Verification items for the finished model (mm, model axes). A direction names the side the tool comes from. Round coordinates to 2 decimals unless told otherwise and drop trailing zeros. Write each loop counter-clockwise with the first axis right and the second up, starting at its lowest first coordinate (ties: lowest second). Pieces come first, ordered by that corner, then holes. Notation, with made-up numbers: (52.5, 89) - (78.5, 89) arc R9 ccw to (78.5, 98) - close; hole circle Ø3 at (20.5, 38). An arc over 180 degrees is marked (long way). Answer as a JSON object with one key per item and string values.
```python
from build123d import *

# Parameters (mm, degrees)
SKETCH_2_W             = 6.925315878
SKETCH_2_H             = 1.1
CUT_EXTRUDE_1_DEPTH    = 11.1
HOLE_WIZARD_M8_1_D     = 6.8
HOLE_WIZARD_M8_1_DEPTH = 19.75
HOLE_WIZARD_M8_1_TIP   = 2.042926105
HOLE_WIZARD_M8_2_D     = 6.8
HOLE_WIZARD_M8_2_DEPTH = 19.75
HOLE_WIZARD_M8_2_TIP   = 2.042926105
CHAMFER_1_SIZE         = 0.2


with BuildPart() as part:
    # 草图1 → 旋转1 (revolve)
    with BuildSketch(Plane.XY):
        Polygon((0, 0), (6, 0), (6, 11.1), (8, 11.1), (8, 13.1), (5, 13.1), (5, 44), (0, 44), align=None)
    revolve(axis=Axis((0, -1000, 0), (0, 1, 0)))

    # 草图2 → 切除-拉伸1 (cut)
    with BuildSketch(Plane.XZ):
        with Locations((0, -5.45)):
            Rectangle(SKETCH_2_W, SKETCH_2_H)
        with Locations((0, 5.45)):
            Rectangle(SKETCH_2_W, SKETCH_2_H)
    extrude(amount=-CUT_EXTRUDE_1_DEPTH, mode=Mode.SUBTRACT)

    # M8 螺纹孔1
    with Locations(Plane(origin=(0, 44, 0), x_dir=(1, 0, 0), z_dir=(0, 1, 0))):
        with Locations((0, 0)):
            Hole(HOLE_WIZARD_M8_1_D / 2, depth=HOLE_WIZARD_M8_1_DEPTH)
            with Locations((0, 0, -(HOLE_WIZARD_M8_1_DEPTH + HOLE_WIZARD_M8_1_TIP / 2))):  # 118° drill point
                Cone(0, HOLE_WIZARD_M8_1_D / 2, HOLE_WIZARD_M8_1_TIP, mode=Mode.SUBTRACT)

    # M8 螺纹孔2
    with Locations(Plane(origin=(0, 0, 0), x_dir=(-1, 0, 0), z_dir=(0, -1, 0))):
        with Locations((0, 0)):
            Hole(HOLE_WIZARD_M8_2_D / 2, depth=HOLE_WIZARD_M8_2_DEPTH)
            with Locations((0, 0, -(HOLE_WIZARD_M8_2_DEPTH + HOLE_WIZARD_M8_2_TIP / 2))):  # 118° drill point
                Cone(0, HOLE_WIZARD_M8_2_D / 2, HOLE_WIZARD_M8_2_TIP, mode=Mode.SUBTRACT)

    # 倒角1
    chamfer_1_edges = [part.edges().sort_by_distance(p)[0] for p in [
        (-5, 44, 0),
    ]]
    chamfer(chamfer_1_edges, length=CHAMFER_1_SIZE)


solid = part.part
```
Q1. Set-up check for faces 1 (the cylindrical face through (-0.74, 10.01, 3.32)), 2 (the flat face through (0, 5, -4.9)), 3 (the cylindrical face through (6, 6, 0)), 4 (the cylindrical face through (-1.08, 28.66, 4.88)): record each of +Z, -Z, +X, -X, +Y, -Y from which the full face is reachable in a straight line by a thin tool's end or side.
Geometry check:
{"face 1": "-Y", "face 2": "-Z, +X, -X, -Y", "face 3": "+X, -Y", "face 4": "+Y"}
Q2. Release check for a two-part mould opening along Z. For faces 5 (the cylindrical face through (0.74, 33.99, 3.32)), 6 (the conical face through (-0.128, 22.562, 0.576)), 7 (the cylindrical face through (-1.73, 12.11, 7.81)), 8 (the flat face through (2, 44, 3)) record: released by +Z, released by -Z, zero draft, split by the parting line, or undercut.
Geometry check:
{"face 5": "undercut", "face 6": "undercut", "face 7": "split by the parting line", "face 8": "zero draft"}
Q3. Section check C-C, the plane y = 29. Record the cut outline in (x, z), then the cut area to 3 significant figures.
Geometry check:
{"outline": "circle Ø10 at (0, 0); hole circle Ø6.8 at (0, 0)", "area": "42.2 mm2"}
Q4. Material ranges on line 1 along Z through (x, y) = (0, 29.5); line 2 along Z through (x, y) = (0, 9); line 3 along Y through (x, z) = (2, 4.75), recorded low to high. Write a range as [from, to].
Geometry check:
{"line 1": "z = [-5, -3.4], [3.4, 5]", "line 2": "z = [-4.9, -3.4], [3.4, 4.9]", "line 3": "y = [0, 13.1]"}
Q5. Section check B-B, the plane z = 6.5. Record the cut outline in (x, y), then the cut area to 3 significant figures.
Geometry check:
{"outline": "(-4.66, 11.1) - (4.66, 11.1) - (4.66, 13.1) - (-4.66, 13.1) - close", "area": "18.7 mm2"}
Q6. Section check A-A, the plane y = 4.5. Record the cut outline in (x, z).
Geometry check:
{"outline": "(-3.46, -4.9) - (3.46, -4.9) arc R6 ccw to (3.46, 4.9) - (-3.46, 4.9) arc R6 ccw to start; hole circle Ø6.8 at (0, 0)"}
Q7. Gauge pin test, flat ends, axial feed: P1, Ø5, axis at x = -3, y = 26.5, coming from the -Z side; P2, Ø6, axis at x = 0, z = 0, coming from the +Y side; P3, Ø2, axis at x = -1.5, y = 3.5, coming from the -Z side. Record the tip position at first contact, or that the pin passes through.
Geometry check:
{"P1": "stops at z = -4.97", "P2": "stops at y = 24.01", "P3": "stops at z = -4.9"}
Q8. Section check D-D, the plane z = -6.25. Record the cut outline in (x, y).
Geometry check:
{"outline": "(-4.99, 11.1) - (4.99, 11.1) - (4.99, 13.1) - (-4.99, 13.1) - close"}
